from build123d import *

# Parameters (mm, degrees)
F3_D = 4


with BuildPart() as f1:
    # F0 (on Front) → F1 (revolve)
    with BuildSketch(Plane.XZ):
        Polygon((-23.5, 20.620037), (-11, 20.620037), (-11, 27.620037), (-22.5, 27.620037), (-22.5, 28.620037), (-23.5, 28.620037), align=None)
    revolve(axis=Axis((0, 0, 24.120037), (0, 0, -1)))

    # F3 (through all)
    with Locations(Plane(origin=(0, 0, 20.620037), x_dir=(1, 0, 0), z_dir=(0, 0, -1))):
        with Locations((-14, 0), (14, 0)):
            Hole(F3_D / 2)


solid = f1.part
Geometry check sheet. Reference: the model listing, model coordinates, mm. A direction names the side the tool comes from. Give positions to 0.01 mm unless a question says otherwise; leave off trailing zeros. Order: outer loops, then holes, each group sorted by start corner. A loop starts at its lowest first (then second) coordinate and runs counter-clockwise, first axis right, second up. Notation, with made-up numbers: (4, -2.5) - (34, -2.5) arc R21 cw to (34, 25.5) - close; hole circle Ø4 at (45.5, -29). An arc over 180 degrees is marked (long way). Answer as a JSON object with one key per item and string values.
(1) Tool access check on faces 4 (the cylindrical face through (2.38, -10.74, 24.17)), 5 (the flat face through (-5, -10, 27.62)). Record the directions out of +Z, -Z, +X, -X, +Y, -Y that give a thin tool (end or side, any length) a straight path to the whole face; none if there is none.
Report:
{"face 4": "+Z, -Z", "face 5": "+Z"}
(2) Cross-section at C-C (z = 26.75). Record the cut outline in (x, y), then the cut area to 3 significant figures.
Report:
{"outline": "circle Ø47 at (0, 0); hole circle Ø4 at (-14, 0); hole circle Ø22 at (0, 0); hole circle Ø4 at (14, 0)", "area": "1,330 mm^2"}
(3) Cross-section at A-A (x = 0). Record the cut outline in (y, z).
Report:
{"outline": "(-23.5, 20.62) - (-11, 20.62) - (-11, 27.62) - (-22.5, 27.62) - (-22.5, 28.62) - (-23.5, 28.62) - close; (11, 20.62) - (23.5, 20.62) - (23.5, 28.62) - (22.5, 28.62) - (22.5, 27.62) - (11, 27.62) - close"}
(4) Depth check by flat-ended pin: pin 1 Ø12 at (x, y) = (-18, -11.5) entering from +Z; pin 2 Ø3 at (x, y) = (-14, 0) entering from +Z; pin 3 Ø1.5 at (x, z) = (-9.5, 26) entering from +Y; pin 4 Ø4.5 at (x, y) = (14, 0) entering from +Z. Enter the tip coordinate at first touch or a pass-through.
Report:
{"pin 1": "z = 28.62", "pin 2": "through", "pin 3": "y = 21.81", "pin 4": "z = 27.62"}
(5) Material ranges on line 1 (Y direction, x = 0, z = 27.25); line 2 (Y direction, x = 14, z = 22.5); line 3 (X direction, y = 9, z = 28), recorded low to high.
Report:
{"line 1": "-23.5 to -11, 11 to 23.5", "line 2": "-18.87 to -2, 2 to 18.87", "line 3": "-21.71 to -20.62, 20.62 to 21.71"}
(6) Draft check along Y on faces 1 (the cylindrical face through (-10.382, -19.961, 28.127)), 2 (the flat face through (23, 0, 28.62)), 3 (the cylindrical face through (-22.4, 7.1, 24.6)). Enter one of: released by +Y, released by -Y, zero draft, split by the parting line, or undercut.
Report:
{"face 1": "undercut", "face 2": "zero draft", "face 3": "split by the parting line"}
(7) Cross-section at B-B (y = -10). Record the cut outline in (x, z).
Report:
{"outline": "(-21.27, 20.62) - (-4.58, 20.62) - (-4.58, 27.62) - (-20.16, 27.62) - (-20.16, 28.62) - (-21.27, 28.62) - close; (4.58, 20.62) - (21.27, 20.62) - (21.27, 28.62) - (20.16, 28.62) - (20.16, 27.62) - (4.58, 27.62) - close"}
